Could you check a few things on this model? Use its own coordinates, in mm. Coordinates: 2 decimals unless noted, no trailing zeros. Loops run counter-clockwise (first coordinate to the right, second up) from the corner with the lowest first, then second, coordinate; pieces in that order, holes last.
1) Imagine slicing it at A-A on z = 1.85. Please give me the cut outline in (x, y).
2) If I drill on line 1 along X through (y, z) = (-3, 2.2); line 2 along X through (y, z) = (-2.5, 4.45); line 3 along Y through (x, z) = (-26, 1.2), over which ranges is the centre line in solid material (lowest first)?
3) Imagine slicing it at C-C on y = -8.25. Please give me the cut outline in (x, z), plus the area to 3 significant figures.
4) Will these pins go through, and if not, where does the flat tip stop? P1, Ø1.8, axis at x = -4.23, y = -2.74, coming from the -Z side; P2, Ø1.5, axis at y = -7.5, z = 4, coming from the +X side.
5) Imagine slicing it at D-D on z = 4.25. Please give me the cut outline in (x, y).
6) Imagine slicing it at B-B on x = -11. Please give me the cut outline in (y, z).
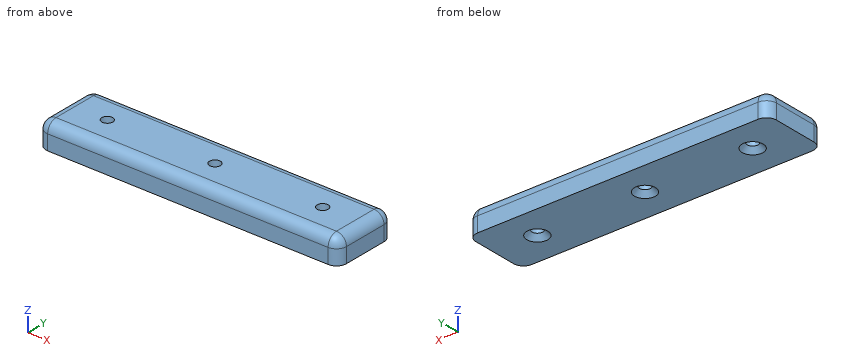
```python
from build123d import *

# Parameters (mm, degrees)
F0_W     = 60
F0_H     = 13
F0_R     = 1.1
F1_DEPTH = 5
F2_R     = 2
F3_SIZE  = 1


with BuildPart() as f1:
    # F0 (on Top) → F1 (new body)
    with BuildSketch(Plane.XY):
        with Locations((-4.228717, -2.739199)):
            Rectangle(F0_W, F0_H)
        with Locations((-25.728717, -2.739199)):
            Circle(F0_R, mode=Mode.SUBTRACT)
        with Locations((-4.228717, -2.739199)):
            Circle(F0_R, mode=Mode.SUBTRACT)
        with Locations((17.271283, -2.739199)):
            Circle(F0_R, mode=Mode.SUBTRACT)
    extrude(amount=F1_DEPTH)

    # F2
    f2_edges = [f1.edges().sort_by_distance(p)[0] for p in [
        (-4.228717, -9.239199, 5),
        (25.771283, -2.739199, 5),
        (25.771283, -9.239199, 2.5),
        (-4.228717, 3.760801, 5),
        (-34.228717, -2.739199, 5),
        (-34.228717, -9.239199, 2.5),
        (25.771283, 3.760801, 2.5),
        (-34.228717, 3.760801, 2.5),
    ]]
    fillet(f2_edges, radius=F2_R)

    # F3
    f3_edges = [f1.edges().sort_by_distance(p)[0] for p in [
        (-5.328717, -2.739199, 0),
        (16.171283, -2.739199, 0),
        (-26.828717, -2.739199, 0),
    ]]
    chamfer(f3_edges, length=F3_SIZE)


solid = f1.part
```
Filled in:
1. outline: (-34.23, -7.24) arc R2 ccw to (-32.23, -9.24) - (23.77, -9.24) arc R2 ccw to (25.77, -7.24) - (25.77, 1.76) arc R2 ccw to (23.77, 3.76) - (-32.23, 3.76) arc R2 ccw to (-34.23, 1.76) - close; hole circle Ø2.2 at (-25.73, -2.74); hole circle Ø2.2 at (-4.23, -2.74); hole circle Ø2.2 at (17.27, -2.74)
2. line 1: x = -34.23 to -26.8, -24.66 to -5.3, -3.16 to 16.2, 18.34 to 25.77
2. line 2: x = -33.61 to -26.8, -24.66 to -5.3, -3.16 to 16.2, 18.34 to 25.15
2. line 3: y = -9.24 to -3.81, -1.67 to 3.76
3. outline: (-33.95, 0) - (25.5, 0) - (25.5, 3) arc R1.73 ccw to (23.77, 4.73) - (-32.23, 4.73) arc R1.73 ccw to (-33.95, 3) - close
3. area: 280 mm2
4. P1: passes through
4. P2: stops at x = 25.75
5. outline: (-33.79, -7.24) arc R1.56 ccw to (-32.23, -8.8) - (23.77, -8.8) arc R1.56 ccw to (25.33, -7.24) - (25.33, 1.76) arc R1.56 ccw to (23.77, 3.32) - (-32.23, 3.32) arc R1.56 ccw to (-33.79, 1.76) - close; hole circle Ø2.2 at (-25.73, -2.74); hole circle Ø2.2 at (-4.23, -2.74); hole circle Ø2.2 at (17.27, -2.74)
6. outline: (-9.24, 0) - (3.76, 0) - (3.76, 3) arc R2 ccw to (1.76, 5) - (-7.24, 5) arc R2 ccw to (-9.24, 3) - close
